```python
from build123d import *

# Parameters (mm, degrees)
BOSS_EXTRUDE1_DEPTH      = 15
BOSS_EXTRUDE1_DEPTH_BACK = 15
SKETCH2_R                = 2.45
BOSS_EXTRUDE2_DEPTH      = 5
CUT_EXTRUDE1_DEPTH       = 31
BOSS_EXTRUDE3_DEPTH      = 25
SKETCH5_W                = 2.662533038
SKETCH5_H                = 5.499463709
CUT_EXTRUDE2_DEPTH       = 3
SKETCH6_W                = 135.823798811
SKETCH6_H                = 59.856144922
CUT_EXTRUDE3_DEPTH       = 46.0000001
SKETCH7_W                = 30
SKETCH7_H                = 30.150652204
CUT_EXTRUDE6_DEPTH       = 139.853804084


with BuildPart() as part:
    # Sketch1 → Boss-Extrude1 (new body, two sides)
    with BuildSketch(Plane.XY) as boss_extrude1_sk:
        with BuildLine():
            Line((-77.5, 0), (77.5, 0))
            ThreePointArc((77.5, 0), (0, 77.5), (-77.5, 0))
        make_face()
    extrude(amount=BOSS_EXTRUDE1_DEPTH)
    extrude(boss_extrude1_sk.sketch, amount=-BOSS_EXTRUDE1_DEPTH_BACK)

    # Sketch2 → Boss-Extrude2 (add)
    with BuildSketch(Plane.XZ):
        with Locations((67.5, 10)):
            Circle(SKETCH2_R)
        with Locations((67.5, -10)):
            Circle(SKETCH2_R)
        with Locations((-67.5, -10)):
            Circle(SKETCH2_R)
        with Locations((-67.5, 10)):
            Circle(SKETCH2_R)
    extrude(amount=BOSS_EXTRUDE2_DEPTH)

    # Sketch3 → Cut-Extrude1 (cut, through all)
    with BuildSketch(Plane.XY.offset(15)):
        with BuildLine():
            Line((-53.909646632, 20), (53.909646632, 20))
            ThreePointArc((53.909646632, 20), (0, -57.5), (-53.909646632, 20))
        make_face()
    extrude(amount=-CUT_EXTRUDE1_DEPTH, mode=Mode.SUBTRACT)

    # Sketch4 → Boss-Extrude3 (add)
    with BuildSketch(Plane(origin=(-77.5, 0, 0), x_dir=(0, 0, -1), z_dir=(1, 0, 0))):
        with BuildLine():
            Line((0, 50), (0, 0))
            Line((0, 0), (30, 0))
            Line((30, 0), (30, 33.846717608))
            ThreePointArc((30, 33.846717608), (17.313763728, 46.220498553), (0, 50))
        make_face()
        with BuildLine():
            Line((-30, 0), (0, 0))
            Line((0, 0), (0, 50))
            ThreePointArc((0, 50), (-17.313763728, 46.220498553), (-30, 33.846717608))
            Line((-30, 33.846717608), (-30, 0))
        make_face()
    extrude(amount=BOSS_EXTRUDE3_DEPTH)

    # Sketch5 → Cut-Extrude2 (cut)
    with BuildSketch(Plane.ZY.offset(77.5)):
        Polygon((-6.086727423, 20.23664057), (-6.086727423, 27.500083204), (-19.368451097, 32.27320265), (-19.368451097, 20.23664057), align=None)
        Polygon((6.086727423, 20.23664057), (6.086727423, 27.500083204), (19.368451097, 32.27320265), (19.368451097, 20.23664057), align=None)
        with BuildLine():
            Line((9.459040074, 11.728036341), (6.086727423, 11.728036341))
            Line((6.086727423, 11.728036341), (6.086727423, 6.228572632))
            Line((6.086727423, 6.228572632), (12.831352726, 6.228572632))
            Line((12.831352726, 6.228572632), (12.831352726, 8.35572369))
            ThreePointArc((12.831352726, 8.35572369), (11.621010767, 10.517694382), (9.459040074, 11.728036341))
        make_face()
        with Locations((1.331266519, 8.978304487)):
            Rectangle(SKETCH5_W, SKETCH5_H)
        with Locations((-1.331266519, 8.978304487)):
            Rectangle(SKETCH5_W, SKETCH5_H)
        with BuildLine():
            ThreePointArc((-9.459040074, 11.728036341), (-11.621010767, 10.517694382), (-12.831352726, 8.35572369))
            Line((-12.831352726, 8.35572369), (-12.831352726, 6.228572632))
            Line((-12.831352726, 6.228572632), (-6.086727423, 6.228572632))
            Line((-6.086727423, 6.228572632), (-6.086727423, 11.728036341))
            Line((-6.086727423, 11.728036341), (-9.459040074, 11.728036341))
        make_face()
    extrude(amount=-CUT_EXTRUDE2_DEPTH, mode=Mode.SUBTRACT)

    # Sketch6 → Cut-Extrude3 (cut, through all)
    with BuildSketch(Plane.XY.offset(15)):
        with Locations((15.411899406, 17.421275335)):
            Rectangle(SKETCH6_W, SKETCH6_H)
    extrude(amount=-CUT_EXTRUDE3_DEPTH, mode=Mode.SUBTRACT)

    # Sketch7 → Cut-Extrude6 (cut, through all)
    with BuildSketch(Plane(origin=(-77.5, 0, 0), x_dir=(0, 0, -1), z_dir=(1, 0, 0))):
        with Locations((0, 62.424673898)):
            Rectangle(SKETCH7_W, SKETCH7_H)
    extrude(amount=CUT_EXTRUDE6_DEPTH, mode=Mode.SUBTRACT)


solid = part.part
```
Verification items for the finished model (mm, model axes). A direction names the side the tool comes from. Give positions to 0.01 mm unless a question says otherwise; leave off trailing zeros. Order: outer loops, then holes, each group sorted by start corner. A loop starts at its lowest first (then second) coordinate and runs counter-clockwise, first axis right, second up. Notation, with made-up numbers: M -9.5,49.5 L 18.5,49.5 A26 cw 18.5,86.5 Z; hole C 29,-26.5 d4. An arc over 180 degrees is marked long. Answer in a Markdown table with one row per item. Add a question column.
Item 1: Section check B-B, the plane y = 23. Enter the section's corners in (x, z).
Item 2: Tool access check on faces 1 (the cylindrical face through (-65.163, -2.465, -9.264)), 2 (the flat face through (-76, 6.229, 9)), 3 (the flat face through (-68, -5, -10)). Record the directions out of +Z, -Z, +X, -X, +Y, -Y that give a thin tool (end or side, any length) a straight path to the whole face; none if there is none.
Item 3: Scan lines: probe 1 along Z at (x, y) = (-56, 45); probe 2 along Y at (x, z) = (-56, -8.5); probe 3 along X at (y, z) = (22, -18). Record each from-to range of solid material in increasing order. Write a range as from..to.
Item 4: Gauge pin test, flat ends, axial feed: pin 1 (4 mm diameter, centred on x = -60, y = 39, fed in from +Z); pin 2 (13 mm diameter, centred on y = 28.5, z = -10, fed in from -X); pin 3 (2 mm diameter, centred on x = -67.5, z = 24, fed in from -Y). Record the tip position at first contact, or that the pin passes through.
Item 5: Mould release check, pull along Y, two halves, no side actions. Record for faces 4 (the flat face through (-68, -5, 10)), 5 (the flat face through (-65, 17, 30)), 6 (the flat face through (-76, 9, 2.663)), 7 (the cylindrical face through (-65.2, 41.7, -23.7)): released by +Y, released by -Y, zero draft, split by the parting line, or undercut.
Item 6: Section check D-D, the plane x = -72. Enter the section's corners in (y, z).
Item 7: Section check A-A, the plane x = -67.5. Enter the section's corners in (y, z), and give its area (3 significant figures).
Item 8: Section check C-C, the plane z = 21.5. Enter the section's corners in (x, y), and give its area (3 significant figures).
Filled sheet:
| question | item | result |
|---|---|---|
| 1 | outline | M -77.5,-30 L -52.5,-30 L -52.5,30 L -77.5,30 L -77.5,19.37 L -74.5,19.37 L -74.5,6.09 L -77.5,6.09 L -77.5,-6.09 L -74.5,-6.09 L -74.5,-19.37 L -77.5,-19.37 Z |
| 2 | face 1 | -Y |
| 2 | face 2 | -X |
| 2 | face 3 | +Z, -Z, +X, -X, -Y |
| 3 | probe 1 | z = -19.39..19.39 |
| 3 | probe 2 | y = 0..47.35 |
| 3 | probe 3 | x = -74.5..-52.5 |
| 4 | pin 1 | stops at z = 27.95 |
| 4 | pin 2 | stops at x = -77.5 |
| 4 | pin 3 | stops at y = 0 |
| 5 | face 4 | released by -Y |
| 5 | face 5 | zero draft |
| 5 | face 6 | undercut |
| 5 | face 7 | released by +Y |
| 6 | outline | M 0,-30 L 33.85,-30 A32.17 ccw 47.35,-15 L 47.35,15 A32.17 ccw 33.85,30 L 0,30 Z |
| 7 | outline | M -5,-12.45 L 0,-12.45 L 0,-30 L 33.85,-30 A32.17 ccw 47.35,-15 L 47.35,15 A32.17 ccw 33.85,30 L 0,30 L 0,12.45 L -5,12.45 L -5,7.55 L 0,7.55 L 0,-7.55 L -5,-7.55 Z |
| 7 | area | 2,730 mm^2 |
| 8 | outline | M -77.5,0 L -52.5,0 L -52.5,43.53 L -77.5,43.53 Z |
| 8 | area | 1,090 mm^2 |
